```python
from build123d import *

# Parameters (mm, degrees)
BOSS_EXTRUDE1_DEPTH = 30
CUT_EXTRUDE1_REACH  = 16.804
SKETCH4_R           = 1.605


with BuildPart() as part:
    # Sketch3 → Boss-Extrude1 (new body)
    with BuildSketch(Plane(origin=(0, 0, 0), x_dir=(0, 0, -1), z_dir=(1, 0, 0))):
        with BuildLine():
            ThreePointArc((47.666821582, 17.564570029), (41.497171662, 29.302299296), (32.5, 39.043437349))
            Line((32.5, 39.043437349), (30.900590551, 37.122008345))
            ThreePointArc((30.900590551, 37.122008345), (39.454988017, 27.860257008), (45.321013433, 16.700171897))
            Line((45.321013433, 16.700171897), (47.666821582, 17.564570029))
        make_face()
        with BuildLine():
            ThreePointArc((30.900590551, 37.122008345), (39.454988017, 27.860257008), (45.321013433, 16.700171897))
            Line((45.321013433, 16.700171897), (30.900590551, 37.122008345))
        make_face()
    extrude(amount=BOSS_EXTRUDE1_DEPTH)

    # Sketch4 → Cut-Extrude1 (cut, up to next)
    with BuildSketch(Plane(origin=(0, 26.911090121, -38.110801992), x_dir=(1, 0, 0), z_dir=(0, -0.576816915, 0.816873458)), mode=Mode.PRIVATE) as cut_extrude1_sk1:
        with Locations((7.75, 0)):
            Circle(SKETCH4_R)
    cut_extrude1_tool1 = extrude(cut_extrude1_sk1.sketch, amount=-CUT_EXTRUDE1_REACH, mode=Mode.PRIVATE) & part.part
    add(cut_extrude1_tool1.solids().sort_by_distance((7.75, 26.91109, -38.110802))[0], mode=Mode.SUBTRACT)
    # Sketch4 → Cut-Extrude1 (cut, up to next)
    with BuildSketch(Plane(origin=(0, 26.911090121, -38.110801992), x_dir=(1, 0, 0), z_dir=(0, -0.576816915, 0.816873458)), mode=Mode.PRIVATE) as cut_extrude1_sk2:
        with Locations((22.25, 0)):
            Circle(SKETCH4_R)
    cut_extrude1_tool2 = extrude(cut_extrude1_sk2.sketch, amount=-CUT_EXTRUDE1_REACH, mode=Mode.PRIVATE) & part.part
    add(cut_extrude1_tool2.solids().sort_by_distance((22.25, 26.91109, -38.110802))[0], mode=Mode.SUBTRACT)


solid = part.part
```
Work out the finished part from the listing and answer in its coordinate system (mm). Round coordinates to 2 decimals unless told otherwise and drop trailing zeros. Loops run counter-clockwise (first coordinate to the right, second up) from the corner with the lowest first, then second, coordinate; pieces in that order, holes last.
(1) The part is cut by section C-C, the plane x = 3.5. Give the vertices of the cut face in (y, z).
Computed values:
outline: (16.7, -45.32) - (17.56, -47.67) arc R50.8 ccw to (39.04, -32.5) - (37.12, -30.9) - close
(2) The part is cut by section B-B, the plane y = 20. Give the vertices of the cut face in (x, z), and give its area (3 significant figures).
Computed values:
outline: (0, -46.7) - (30, -46.7) - (30, -42.99) - (0, -42.99) - close
area: 111 mm2
(3) Each of these flat-tipped pins is pushed along its axis until it touches: P1, Ø10, axis at x = 12, y = 31.5, coming from the -Z side; P2, Ø2, axis at x = 13, y = 30, coming from the -Z side; P3, Ø1, axis at x = 26, y = 25, coming from the -Z side; P4, Ø3, axis at y = 27.5, z = -35.5, coming from the +X side. Where does it stop, or does it pass through?
Computed values:
P1: stops at z = -43.34
P2: stops at z = -41.71
P3: stops at z = -44.5
P4: passes through
(4) The mould has two halves that part along Y. Classify faces 1 (the cylindrical face through (8.61, 29.2, -39)), 2 (the cylindrical face through (14.79, 29.15, -41.604)), 3 (the flat face through (0, 28, -40)): pulls with the +Y half, pulls with the -Y half, needs draft (parallel to the pull), parting line crosses it, or undercut.
Computed values:
face 1: undercut
face 2: pulls with the +Y half
face 3: needs draft
(5) The part is cut by section D-D, the plane z = -40. Give the number of separate pieces and of enclosed holes in the cut face, and give its area (3 significant figures).
Computed values:
separate pieces: 1
enclosed holes: 2
area: 193 mm2
(6) Find the intervals of material crossed by L1, parallel to Y at x = 21, z = -37.5; L2, parallel to Y at x = 23, z = -44.25; L3, parallel to Z at x = 5, y = 20.25, in increasing order.
Computed values:
L1: y = 27.78 to 34.27
L2: y = 18.22 to 24.95
L3: z = -46.59 to -42.81
(7) The part is cut by section A-A, the plane x = 21. Give the vertices of the cut face in (y, z).
Computed values:
outline: (16.7, -45.32) - (17.56, -47.67) arc R50.8 ccw to (28.47, -42.07) - (26.09, -38.69) - close; (27.73, -37.53) - (30.12, -40.91) arc R50.8 ccw to (39.04, -32.5) - (37.12, -30.9) - close
